Here's how the part is built. I have some questions about the finished solid (model axes, mm). Round coordinates to 2 decimals unless told otherwise and drop trailing zeros. Write each loop counter-clockwise with the first axis right and the second up, starting at its lowest first coordinate (ties: lowest second). Pieces come first, ordered by that corner, then holes. Notation, with made-up numbers: M 38.25,84.5 L 43.25,84.5 A23 ccw 43.25,97.5 Z; hole C 37,78 d11. An arc over 180 degrees is marked long. Write item = value, one per line. Start each with the question number.
(1) I want a section at A-A (y = -10.5). List the corners of the cut face in (x, z) for me, and give its area (3 significant figures).
(2) I want a section at D-D (x = 50). List the corners of the cut face in (y, z) for me.
(3) I need wall thicknesses on line 1 along Y through (x, z) = (-36.5, 0.8); line 2 along X through (y, z) = (19.5, 0.8); line 3 along Y through (x, z) = (35.5, 1.85). Which ranges of each line are inside material? Lowest first, please.
(4) I want a section at C-C (x = -9). List the corners of the cut face in (y, z) for me, and give its area (3 significant figures).
(5) I want a section at B-B (z = 0.35). List the corners of the cut face in (x, y) for me, and give its area (3 significant figures).
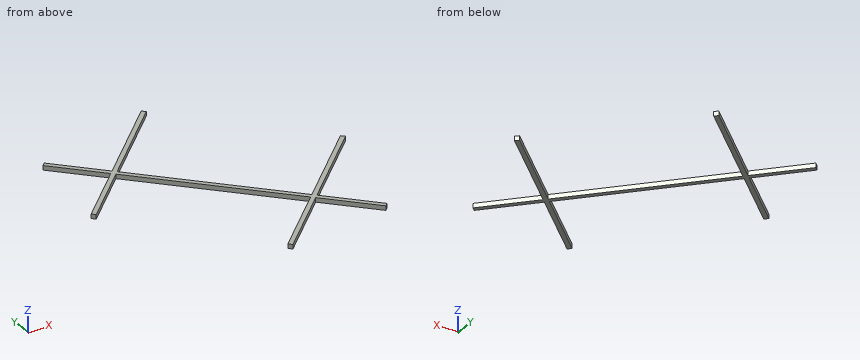
Autodesk Inventor part; units mm, degrees
ref_plane "YZ Plane" through (0, 0, 0) normal (1, 0, 0) x (0, 1, 0)
ref_plane "XZ Plane" through (0, 0, 0) normal (0, 1, 0) x (-1, 0, 0)
ref_plane "XY Plane" through (0, 0, 0) normal (0, 0, 1) x (1, 0, 0)
sketch "Sketch1" plane through (0, 0, 0) normal (0, 0, 1) x (1, 0, 0)
  arc A0 (5.5811, -56.8606) -> (20.209, -64.6836) centre (38.8796, -12.1848) ccw construction
  arc A1 (-7.6539, -43.4667) -> (5.5811, -56.8606) centre (37.8873, -11.7018) ccw construction
  arc A2 (-7.6539, -43.4667) -> (-31.2183, -12.0793) centre (-386.265, -303.1724) ccw construction
  arc A3 (-31.2183, -12.0793) -> (-63.3277, 19.0744) centre (-191.6112, -145.2692) ccw construction
  arc A4 (-67.5206, 26.3221) -> (-63.3277, 19.0744) centre (-54.6162, 28.9507) ccw construction
  arc A5 (-66.9469, 41.0059) -> (-67.5206, 26.3221) centre (-15.6776, 31.6496) ccw construction
  line L0 (-66.9469, 41.0059) -> (-26.0985, 81.0785) construction
  arc A6 (-3.6955, 79.7027) -> (-26.0985, 81.0785) centre (-17.6076, 36.2535) ccw construction
  arc A7 (1.4491, 74.6716) -> (-3.6955, 79.7027) centre (-6.1453, 72.0517) ccw construction
  arc A8 (2.6831, 69.1533) -> (1.4491, 74.6716) centre (-18.5892, 67.2935) ccw construction
  arc A9 (2.6831, 69.1533) -> (3.1898, 63.5624) centre (229.5421, 86.8959) ccw construction
  arc A10 (3.1898, 63.5624) -> (8.7161, 49.818) centre (30.4167, 66.5265) ccw construction
  arc A11 (8.7161, 49.818) -> (19.0471, 39.3259) centre (47.1297, 77.3097) ccw construction
  arc A12 (19.0471, 39.3259) -> (32.6891, 29.8296) centre (104.4845, 147.5139) ccw construction
  arc A13 (32.6891, 29.8296) -> (50.5655, 19.6706) centre (502.3948, 835.5524) ccw construction
  arc A14 (57.8671, 12.5741) -> (50.5655, 19.6706) centre (33.0101, -5.6965) ccw construction
  arc A15 (67.0572, -4.125) -> (57.8671, 12.5741) centre (18.4686, -19.9867) ccw construction
  arc A16 (68.9532, -23.0115) -> (67.0572, -4.125) centre (24.8632, -17.8992) ccw construction
  line L1 (-52.1723, 55.4999) -> (42.0363, -41.3708)
  line L2 (43.4701, -39.9764) -> (-50.7446, 56.9005)
  line L3 (42.0363, -41.3708) -> (43.4701, -39.9764)
  line L4 (-4.1456, -47.7345) -> (58.0182, 12.7211)
  line L5 (56.6239, 14.1548) -> (-5.54, -46.3007)
  line L6 (-55.3767, 12.3052) -> (3.7843, 69.8404)
  line L7 (2.3899, 71.2742) -> (-56.7711, 13.739)
  line L8 (-56.7711, 13.739) -> (-55.3767, 12.3052)
  line L9 (2.3899, 71.2742) -> (3.7843, 69.8404)
  line L10 (-52.1723, 55.4999) -> (-50.7446, 56.9005)
  line L11 (-4.1456, -47.7345) -> (-5.54, -46.3007)
  line L12 (58.0182, 12.7211) -> (56.6239, 14.1548)
  point P0 (0, 0)
  point P1 (-8.2693, 4.2237)
  point P2 (-4.9861, 4.7501)
  point P3 (-66.0155, 22.3561)
  point P4 (24.203, -20.1649)
  point P5 (22.8086, -18.7311)
  point P6 (-30.7071, 36.2969)
  point P7 (-32.1015, 37.7306)
  point P8 (-33.5353, 36.3363)
  point P9 (-32.1409, 34.9025)
  point P10 (21.3749, -20.1255)
  point P11 (22.7692, -21.5593)
  dimension "d243" = 2
  dimension "d244" = 2
  dimension "d245" = 2
extrude "Extrusion12" add sketch "Sketch1" along normal blind 2
properties part number "print008_Grundform_innen_neu"
Returned:
q1.outline = M 12.01,0 L 14.8,0 L 14.8,2 L 12.01,2 Z; M 31.27,0 L 34.14,0 L 34.14,2 L 31.27,2 Z
q1.area = 11.3 mm²
q2.outline = M 4.92,0 L 7.71,0 L 7.71,2 L 4.92,2 Z
q3.line_1 = 30.66 to 33.45, 39.38 to 42.25
q3.line_2 = -50.85 to -47.98, -17.16 to -14.37
q3.line_3 = -34.65 to -31.78, -9.18 to -6.39
q4.outline = M 11.11,0 L 13.98,0 L 13.98,2 L 11.11,2 Z; M 57.41,0 L 60.2,0 L 60.2,2 L 57.41,2 Z
q4.area = 11.3 mm²
q5.outline = M -56.77,13.74 L -55.38,12.31 L -32.14,34.9 L 21.37,-20.13 L -5.54,-46.3 L -4.15,-47.73 L 22.77,-21.56 L 42.04,-41.37 L 43.47,-39.98 L 24.2,-20.16 L 58.02,12.72 L 56.62,14.15 L 22.81,-18.73 L -30.71,36.3 L 3.78,69.84 L 2.39,71.27 L -32.1,37.73 L -50.74,56.9 L -52.17,55.5 L -33.54,36.34 Z
q5.area = 601 mm²
